from build123d import *

# Parameters (mm, degrees)
SKETCH_2_W          = 60
SKETCH_2_H          = 20
EXTRUDE_1_DEPTH     = 180
SKETCH_14_W         = 20
SKETCH_14_H         = 125
CUT_EXTRUDE_1_DEPTH = 184.575597507
FILLET_1_R          = 5


with BuildPart() as part:
    # 草圖2 → 填料-伸長1 (new body)
    with BuildSketch(Plane.XY):
        Rectangle(SKETCH_2_W, SKETCH_2_H)
    extrude(amount=-EXTRUDE_1_DEPTH)

    # 草圖14 → 除料-伸長1 (cut, through all)
    with BuildSketch(Plane(origin=(0, 10, 0), x_dir=(1, 0, 0), z_dir=(0, 1, 0))):
        with Locations((0, 92.5)):
            Rectangle(SKETCH_14_W, SKETCH_14_H)
    extrude(amount=-CUT_EXTRUDE_1_DEPTH, mode=Mode.SUBTRACT)

    # 圓角1
    fillet_1_edges = [part.edges().sort_by_distance(p)[0] for p in [
        (10, 10, -92.5),
        (-10, 10, -92.5),
    ]]
    fillet(fillet_1_edges, radius=FILLET_1_R)


solid = part.part
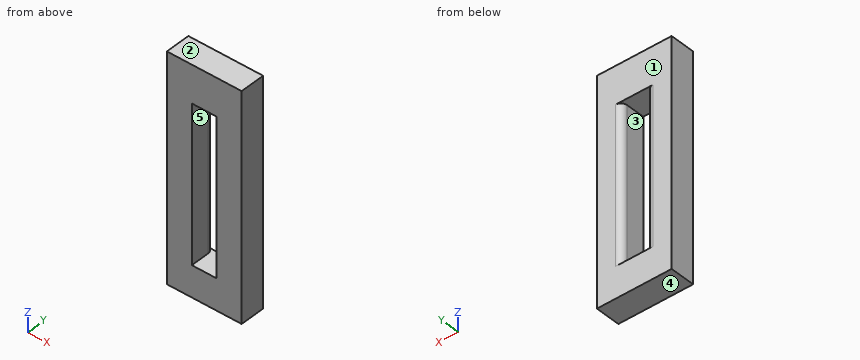
Can you work these out from the model? Positions are in its coordinate system, mm. Face numbers are marked on the shaded views. A direction names the side the tool comes from. Round coordinates to 2 decimals unless told otherwise and drop trailing zeros. Write each loop counter-clockwise with the first axis right and the second up, starting at its lowest first coordinate (ties: lowest second). Pieces come first, ordered by that corner, then holes. Notation, with made-up numbers: (15.25, -18) -> (22.25, -18) arc R20 cw to (22.25, 20) -> close; hole circle Ø11 at (24.5, 50). An arc over 180 degrees is marked (long way). One line per question, with ' | ' between items. Start each with the question number.
1) Suppose I cut it at C-C on y = -6.75. Write out the boundary of the cut face in (x, z).
2) Suppose I cut it at B-B on x = -2. Write out the boundary of the cut face in (y, z).
3) I'm going to push a flat-ended pin straight in: P1, Ø10, axis at x = 10.5, y = -6.5, coming from the +Z side. Where does the tip first touch, or does it pass through?
4) I need wall thicknesses on line 1 (Z direction, x = 9.5, y = -5); line 2 (X direction, y = -6, z = -51.5); line 3 (Y direction, x = -13, z = -59). Which ranges of each line are inside material? Lowest first, please. Write a range as [from, to].
5) Suppose I cut it at D-D on x = -12. Write out the boundary of the cut face in (y, z).
6) Suppose I cut it at A-A on z = -67.5. Write out the boundary of the cut face in (x, y).
7) If we mould it in two halves opening along Z, with no side actions, what happens to the marked faces 1, 2 and 3? For each: released by +Z, released by -Z, zero draft, split by the parting line, or undercut.
8) On a 3-axis mill with a long thin cutter (end or side, diameter ignored), from which of +Z, -Z, +X, -X, +Y, -Y can I reach the whole of each face in a straight line? I mean the marked faces 4 and 5. Say none if no direction works.
Return value:
1) outline: (-30, -180) -> (30, -180) -> (30, 0) -> (-30, 0) -> close; hole (-10, -155) -> (10, -155) -> (10, -30) -> (-10, -30) -> close
2) outline: (-10, -180) -> (10, -180) -> (10, -155) -> (-10, -155) -> close; (-10, -30) -> (10, -30) -> (10, 0) -> (-10, 0) -> close
3) P1: stops at z = 0
4) line 1: z = [-180, -155], [-30, 0] | line 2: x = [-30, -10], [10, 30] | line 3: y = [-10, 9.58]
5) outline: (-10, -180) -> (10, -180) -> (10, -155) -> (9, -155) -> (9, -30) -> (10, -30) -> (10, 0) -> (-10, 0) -> close
6) outline: (-30, -10) -> (-10, -10) -> (-10, 5) arc R5 ccw to (-15, 10) -> (-30, 10) -> close; (10, -10) -> (30, -10) -> (30, 10) -> (15, 10) arc R5 ccw to (10, 5) -> close
7) face 1: zero draft | face 2: released by +Z | face 3: undercut
8) face 4: -Z, +X, -X, +Y, -Y | face 5: +Y, -Y
